Work out the finished part from the listing and answer in its coordinate system (mm). Round coordinates to 2 decimals unless told otherwise and drop trailing zeros. Order: outer loops, then holes, each group sorted by start corner. A loop starts at its lowest first (then second) coordinate and runs counter-clockwise, first axis right, second up. Notation, with made-up numbers: M 53.5,-14.5 L 99.5,-14.5 A13 ccw 99.5,0.5 Z; hole C 65,12.25 d11. An arc over 180 degrees is marked long. Return JSON: item names as keys, results as strings.
from build123d import *

# Parameters (mm, degrees)
SKETCH1_W           = 160
SKETCH1_H           = 35
SKETCH1_R           = 1.25
SKETCH1_R_2         = 4
BOSS_EXTRUDE1_DEPTH = 3
SKETCH3_R           = 1.25
CUT_EXTRUDE7_DEPTH  = 10


with BuildPart() as part:
    # Sketch1 → Boss-Extrude1 (new body)
    with BuildSketch(Plane(origin=(0, 0, 0), x_dir=(1, 0, 0), z_dir=(0, 1, 0))):
        with Locations((-20, 5)):
            Rectangle(SKETCH1_W, SKETCH1_H)
        with Locations((-97, -9.5)):
            Circle(SKETCH1_R, mode=Mode.SUBTRACT)
        with Locations((-97, -3)):
            Circle(SKETCH1_R, mode=Mode.SUBTRACT)
        with Locations((-88.75, 1)):
            Circle(SKETCH1_R, mode=Mode.SUBTRACT)
        with Locations((-61.25, 1)):
            Circle(SKETCH1_R, mode=Mode.SUBTRACT)
        with Locations((-88.75, 8)):
            Circle(SKETCH1_R, mode=Mode.SUBTRACT)
        with Locations((-61.25, 8)):
            Circle(SKETCH1_R, mode=Mode.SUBTRACT)
        with Locations((-2, 5)):
            Circle(SKETCH1_R, mode=Mode.SUBTRACT)
        with Locations((25, 5)):
            Circle(SKETCH1_R_2, mode=Mode.SUBTRACT)
        with Locations((52, 5)):
            Circle(SKETCH1_R, mode=Mode.SUBTRACT)
    extrude(amount=BOSS_EXTRUDE1_DEPTH)

    # Sketch3 → Cut-Extrude7 (cut)
    with BuildSketch(Plane(origin=(0, 3, 0), x_dir=(-1, 0, 0), z_dir=(0, -1, 0))):
        with Locations((-44, -9.307637977)):
            Circle(SKETCH3_R)
        with Locations((-44, 19.692362023)):
            Circle(SKETCH3_R)
        with Locations((-6, 19.692362023)):
            Circle(SKETCH3_R)
        with Locations((-6, -9.307637977)):
            Circle(SKETCH3_R)
    extrude(amount=CUT_EXTRUDE7_DEPTH, mode=Mode.SUBTRACT)


solid = part.part
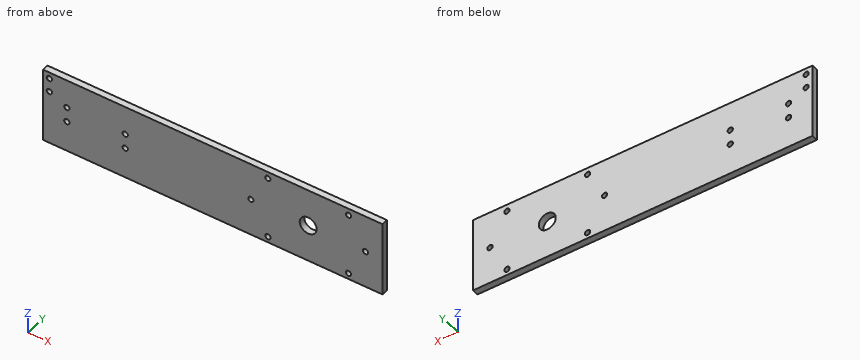
Item 1: Each of these flat-tipped pins is pushed along its axis until it touches: pin 1 (1.5 mm diameter, centred on x = -88.75, z = -1, fed in from +Y); pin 2 (1 mm diameter, centred on x = 20, z = 1.5, fed in from -Y). Where does it stop, or does it pass through?
Output:
{"pin 1": "passes through", "pin 2": "stops at y = 0"}
Item 2: Consider line 1 along X through (y, z) = (2.35, 9.5); line 2 along X through (y, z) = (1.35, -5); line 3 along Z through (x, y) = (44, 2.35). Determine where each line is inside the solid, lowest interval first. Write a range as [from, to].
Output:
{"line 1": "x = [-100, -98.25], [-95.75, 4.76], [7.24, 42.76], [45.24, 60]", "line 2": "x = [-100, -3.25], [-0.75, 21], [29, 50.75], [53.25, 60]", "line 3": "z = [-22.5, -20.94], [-18.44, 8.06], [10.56, 12.5]"}
Item 3: Find section A-A (x = 25). Determine the outline of the cut face in (y, z), plus the area to 3 significant figures.
Output:
{"outline": "M 0,-22.5 L 3,-22.5 L 3,-9 L 0,-9 Z; M 0,-1 L 3,-1 L 3,12.5 L 0,12.5 Z", "area": "81.0 mm^2"}
Item 4: Find section B-B (y = 1.95). State how many separate pieces and enclosed holes the cut face has, plus the area to 3 significant figures.
Output:
{"separate pieces": "1", "enclosed holes": "13", "area": "5,490 mm^2"}
